The listing builds one solid part. Answer for the finished solid, in the listing's coordinates (mm). A direction names the side the tool comes from. Give positions to 0.01 mm unless a question says otherwise; leave off trailing zeros. Write each loop counter-clockwise with the first axis right and the second up, starting at its lowest first coordinate (ties: lowest second). Pieces come first, ordered by that corner, then holes. Notation, with made-up numbers: (-7, 25.5) - (23, 25.5) arc R10 cw to (23, 34.5) - close; hole circle Ø11 at (78, 6). An arc over 180 degrees is marked (long way). Answer as CSV lines item,"result". Start each with the question number.
(1) Straight lines are drawn through the part: probe 1 along Y at (x, z) = (4, 0.8); probe 2 along Y at (x, z) = (20.6, 27); probe 3 along Z at (x, y) = (21.25, -32.5). For each, find the intervals that lie inside material, in ascending order.
(2) Find section D-D (x = 6.25). Write down the section's boundary in (y, z).
(3) Find section B-B (x = 16). Write down the section's boundary in (y, z).
(4) Each of these flat-tipped pins is pushed along its axis until it touches: pin 1 Ø2 at (x, y) = (17, -13.5) entering from -Z; pin 2 Ø3.5 at (y, z) = (-11.89, 16.39) entering from -X. Where does it stop, or does it pass through?
(5) Find section A-A (z = 12). Write down the section's boundary in (x, y).
(6) Find section C-C (y = -19). Write down the section's boundary in (x, z).
(7) For faces 1 (the face through (0, -23, 1)), 2 (the face through (15, -15, 1.999)), determine the directions among +Z, -Z, +X, -X, +Y, -Y from which every point of the face is accessible in a straight line to the end or side of a thin tool.
(8) For a pull along Y with two mould halves and no side action, classify faces 3 (the face through (19, -23, 39)), 4 (the face through (5.386, -14.075, 1.014)) as pulls with the +Y half, pulls with the -Y half, needs draft (parallel to the pull), parting line crosses it, or undercut.
from build123d import *

# Parameters (mm, degrees)
SKETCH_1_W               = 22.5
SKETCH_1_H               = 45
EXTRUDE_1_DEPTH          = 2
SKETCH_2_W               = 3.5
SKETCH_2_H               = 45
EXTRUDE_2_DEPTH          = 52
CUT_EXTRUDE_2_REACH      = 24.5
SKETCH_3_R               = 2.1
SKETCH_3_R_2             = 11.5
SKETCH_3_R_3             = 1.5
CHAMFER_1_SIZE           = 6
CHAMFER_1_SIZE2          = 2
FILLET_1_R               = 1
SKETCH_4_R               = 1.5
CUT_EXTRUDE_3_DEPTH      = 5
SKETCH_5_R               = 2.24713436
CUT_EXTRUDE_4_DEPTH      = 15
CUT_EXTRUDE_4_DEPTH_BACK = 0.001


with BuildPart() as part:
    # 草图1 → 凸台-拉伸1 (new body)
    with BuildSketch(Plane.XY):
        with Locations((11.25, -22.5)):
            Rectangle(SKETCH_1_W, SKETCH_1_H)
    extrude(amount=EXTRUDE_1_DEPTH)

    # 草图2 → 凸台-拉伸2 (add)
    with BuildSketch(Plane.XY.offset(2)):
        with Locations((20.75, -22.5)):
            Rectangle(SKETCH_2_W, SKETCH_2_H)
    extrude(amount=EXTRUDE_2_DEPTH)

    # 草图3 → 切除-拉伸2 (cut, up to next)
    with BuildSketch(Plane(origin=(22.5, 0, 0), x_dir=(0, 0, -1), z_dir=(1, 0, 0)), mode=Mode.PRIVATE) as cut_extrude_2_sk1:
        with Locations((-46.97375327, -5.855205609)):
            Circle(SKETCH_3_R)
    cut_extrude_2_tool1 = extrude(cut_extrude_2_sk1.sketch, amount=-CUT_EXTRUDE_2_REACH, mode=Mode.PRIVATE) & part.part
    add(cut_extrude_2_tool1.solids().sort_by_distance((22.5, -5.855206, 46.973753))[0], mode=Mode.SUBTRACT)
    # 草图3 → 切除-拉伸2 (cut, up to next)
    with BuildSketch(Plane(origin=(22.5, 0, 0), x_dir=(0, 0, -1), z_dir=(1, 0, 0)), mode=Mode.PRIVATE) as cut_extrude_2_sk2:
        with Locations((-7.02624673, -39.144794391)):
            Circle(SKETCH_3_R)
    cut_extrude_2_tool2 = extrude(cut_extrude_2_sk2.sketch, amount=-CUT_EXTRUDE_2_REACH, mode=Mode.PRIVATE) & part.part
    add(cut_extrude_2_tool2.solids().sort_by_distance((22.5, -39.144794, 7.026247))[0], mode=Mode.SUBTRACT)
    # 草图3 → 切除-拉伸2 (cut, up to next)
    with BuildSketch(Plane(origin=(22.5, 0, 0), x_dir=(0, 0, -1), z_dir=(1, 0, 0)), mode=Mode.PRIVATE) as cut_extrude_2_sk3:
        with Locations((-27, -22.5)):
            Circle(SKETCH_3_R_2)
    cut_extrude_2_tool3 = extrude(cut_extrude_2_sk3.sketch, amount=-CUT_EXTRUDE_2_REACH, mode=Mode.PRIVATE) & part.part
    add(cut_extrude_2_tool3.solids().sort_by_distance((22.5, -22.5, 27))[0], mode=Mode.SUBTRACT)
    # 草图3 → 切除-拉伸2 (cut, up to next)
    with BuildSketch(Plane(origin=(22.5, 0, 0), x_dir=(0, 0, -1), z_dir=(1, 0, 0)), mode=Mode.PRIVATE) as cut_extrude_2_sk4:
        with Locations((-46.97375327, -39.144794391)):
            Circle(SKETCH_3_R)
    cut_extrude_2_tool4 = extrude(cut_extrude_2_sk4.sketch, amount=-CUT_EXTRUDE_2_REACH, mode=Mode.PRIVATE) & part.part
    add(cut_extrude_2_tool4.solids().sort_by_distance((22.5, -39.144794, 46.973753))[0], mode=Mode.SUBTRACT)
    # 草图3 → 切除-拉伸2 (cut, up to next)
    with BuildSketch(Plane(origin=(22.5, 0, 0), x_dir=(0, 0, -1), z_dir=(1, 0, 0)), mode=Mode.PRIVATE) as cut_extrude_2_sk5:
        with Locations((-7.02624673, -5.855205609)):
            Circle(SKETCH_3_R)
    cut_extrude_2_tool5 = extrude(cut_extrude_2_sk5.sketch, amount=-CUT_EXTRUDE_2_REACH, mode=Mode.PRIVATE) & part.part
    add(cut_extrude_2_tool5.solids().sort_by_distance((22.5, -5.855206, 7.026247))[0], mode=Mode.SUBTRACT)
    # 草图3 → 切除-拉伸2 (cut, up to next)
    with BuildSketch(Plane(origin=(22.5, 0, 0), x_dir=(0, 0, -1), z_dir=(1, 0, 0)), mode=Mode.PRIVATE) as cut_extrude_2_sk6:
        with Locations((-42, -22.5)):
            Circle(SKETCH_3_R_3)
    cut_extrude_2_tool6 = extrude(cut_extrude_2_sk6.sketch, amount=-CUT_EXTRUDE_2_REACH, mode=Mode.PRIVATE) & part.part
    add(cut_extrude_2_tool6.solids().sort_by_distance((22.5, -22.5, 42))[0], mode=Mode.SUBTRACT)
    # 草图3 → 切除-拉伸2 (cut, up to next)
    with BuildSketch(Plane(origin=(22.5, 0, 0), x_dir=(0, 0, -1), z_dir=(1, 0, 0)), mode=Mode.PRIVATE) as cut_extrude_2_sk7:
        with Locations((-37.606601718, -11.893398282)):
            Circle(SKETCH_3_R_3)
    cut_extrude_2_tool7 = extrude(cut_extrude_2_sk7.sketch, amount=-CUT_EXTRUDE_2_REACH, mode=Mode.PRIVATE) & part.part
    add(cut_extrude_2_tool7.solids().sort_by_distance((22.5, -11.893398, 37.606602))[0], mode=Mode.SUBTRACT)
    # 草图3 → 切除-拉伸2 (cut, up to next)
    with BuildSketch(Plane(origin=(22.5, 0, 0), x_dir=(0, 0, -1), z_dir=(1, 0, 0)), mode=Mode.PRIVATE) as cut_extrude_2_sk8:
        with Locations((-27, -7.5)):
            Circle(SKETCH_3_R_3)
    cut_extrude_2_tool8 = extrude(cut_extrude_2_sk8.sketch, amount=-CUT_EXTRUDE_2_REACH, mode=Mode.PRIVATE) & part.part
    add(cut_extrude_2_tool8.solids().sort_by_distance((22.5, -7.5, 27))[0], mode=Mode.SUBTRACT)
    # 草图3 → 切除-拉伸2 (cut, up to next)
    with BuildSketch(Plane(origin=(22.5, 0, 0), x_dir=(0, 0, -1), z_dir=(1, 0, 0)), mode=Mode.PRIVATE) as cut_extrude_2_sk9:
        with Locations((-16.393398282, -11.893398282)):
            Circle(SKETCH_3_R_3)
    cut_extrude_2_tool9 = extrude(cut_extrude_2_sk9.sketch, amount=-CUT_EXTRUDE_2_REACH, mode=Mode.PRIVATE) & part.part
    add(cut_extrude_2_tool9.solids().sort_by_distance((22.5, -11.893398, 16.393398))[0], mode=Mode.SUBTRACT)
    # 草图3 → 切除-拉伸2 (cut, up to next)
    with BuildSketch(Plane(origin=(22.5, 0, 0), x_dir=(0, 0, -1), z_dir=(1, 0, 0)), mode=Mode.PRIVATE) as cut_extrude_2_sk10:
        with Locations((-12, -22.5)):
            Circle(SKETCH_3_R_3)
    cut_extrude_2_tool10 = extrude(cut_extrude_2_sk10.sketch, amount=-CUT_EXTRUDE_2_REACH, mode=Mode.PRIVATE) & part.part
    add(cut_extrude_2_tool10.solids().sort_by_distance((22.5, -22.5, 12))[0], mode=Mode.SUBTRACT)
    # 草图3 → 切除-拉伸2 (cut, up to next)
    with BuildSketch(Plane(origin=(22.5, 0, 0), x_dir=(0, 0, -1), z_dir=(1, 0, 0)), mode=Mode.PRIVATE) as cut_extrude_2_sk11:
        with Locations((-16.393398282, -33.106601718)):
            Circle(SKETCH_3_R_3)
    cut_extrude_2_tool11 = extrude(cut_extrude_2_sk11.sketch, amount=-CUT_EXTRUDE_2_REACH, mode=Mode.PRIVATE) & part.part
    add(cut_extrude_2_tool11.solids().sort_by_distance((22.5, -33.106602, 16.393398))[0], mode=Mode.SUBTRACT)
    # 草图3 → 切除-拉伸2 (cut, up to next)
    with BuildSketch(Plane(origin=(22.5, 0, 0), x_dir=(0, 0, -1), z_dir=(1, 0, 0)), mode=Mode.PRIVATE) as cut_extrude_2_sk12:
        with Locations((-27, -37.5)):
            Circle(SKETCH_3_R_3)
    cut_extrude_2_tool12 = extrude(cut_extrude_2_sk12.sketch, amount=-CUT_EXTRUDE_2_REACH, mode=Mode.PRIVATE) & part.part
    add(cut_extrude_2_tool12.solids().sort_by_distance((22.5, -37.5, 27))[0], mode=Mode.SUBTRACT)
    # 草图3 → 切除-拉伸2 (cut, up to next)
    with BuildSketch(Plane(origin=(22.5, 0, 0), x_dir=(0, 0, -1), z_dir=(1, 0, 0)), mode=Mode.PRIVATE) as cut_extrude_2_sk13:
        with Locations((-37.606601718, -33.106601718)):
            Circle(SKETCH_3_R_3)
    cut_extrude_2_tool13 = extrude(cut_extrude_2_sk13.sketch, amount=-CUT_EXTRUDE_2_REACH, mode=Mode.PRIVATE) & part.part
    add(cut_extrude_2_tool13.solids().sort_by_distance((22.5, -33.106602, 37.606602))[0], mode=Mode.SUBTRACT)

    # 倒角1
    chamfer_1_edges = [part.edges().sort_by_distance(p)[0] for p in [
        (19, -22.5, 2),
    ]]
    chamfer_1_side = [part.faces().sort_by_distance(p)[0] for p in [
        (9.5, -22.5, 2),
    ]]
    chamfer(chamfer_1_edges, length=CHAMFER_1_SIZE, length2=CHAMFER_1_SIZE2, reference=chamfer_1_side[0])

    # 圆角1
    fillet_1_edges = [part.edges().sort_by_distance(p)[0] for p in [
        (20.75, 0, 54),
        (19, -22.5, 54),
        (20.75, -45, 54),
        (22.5, -22.5, 54),
    ]]
    fillet(fillet_1_edges, radius=FILLET_1_R)

    # 草图4 → 切除-拉伸3 (cut, symmetric)
    with BuildSketch(Plane.XY.offset(2)):
        with Locations((4, -31.5)):
            Circle(SKETCH_4_R)
        with Locations((4, -13.5)):
            Circle(SKETCH_4_R)
        with Locations((16, -13.5)):
            Circle(SKETCH_4_R)
        with Locations((16, -31.5)):
            Circle(SKETCH_4_R)
    extrude(amount=CUT_EXTRUDE_3_DEPTH, both=True, mode=Mode.SUBTRACT)

    # 草图5 → 切除-拉伸4 (cut, two sides)
    with BuildSketch(Plane.XY.offset(2)) as cut_extrude_4_sk:
        with Locations((16, -13.5)):
            Circle(SKETCH_5_R)
        with Locations((16, -31.5)):
            Circle(SKETCH_5_R)
    extrude(amount=CUT_EXTRUDE_4_DEPTH, mode=Mode.SUBTRACT)
    extrude(cut_extrude_4_sk.sketch, amount=-CUT_EXTRUDE_4_DEPTH_BACK, mode=Mode.SUBTRACT)


solid = part.part
Result set:
1,probe 1,"-45 to -33, -30 to -15, -12 to 0"
1,probe 2,"-45 to -39, -36 to -34, -11 to -9, -6 to 0"
1,probe 3,"0 to 15.02, 17.77 to 21.32, 32.68 to 36.23, 38.98 to 54"
2,outline,"(-45, 0) - (0, 0) - (0, 2) - (-45, 2) - close"
3,outline,"(-45, 0) - (-33, 0) - (-33, 2) - (-33.75, 2) - (-33.75, 3) - (-45, 3) - close; (-30, 0) - (-15, 0) - (-15, 2) - (-15.75, 2) - (-15.75, 3) - (-29.25, 3) - (-29.25, 2) - (-30, 2) - close; (-12, 0) - (0, 0) - (0, 3) - (-11.25, 3) - (-11.25, 2) - (-12, 2) - close"
4,pin 1,"z = 0"
4,pin 2,"x = 19"
5,outline,"(19, -45) - (22.5, -45) - (22.5, -24) - (19, -24) - close; (19, -21) - (22.5, -21) - (22.5, 0) - (19, 0) - close"
6,outline,"(0, 0) - (22.5, 0) - (22.5, 16.05) - (19, 16.05) - (19, 4) - (13, 2) - (0, 2) - close; (19, 37.95) - (22.5, 37.95) - (22.5, 53) arc R1 ccw to (21.5, 54) - (20, 54) arc R1 ccw to (19, 53) - close"
7,face 1,"+Z, -Z, -X, +Y, -Y"
7,face 2,"+Z"
8,face 3,"needs draft"
8,face 4,"undercut"
